Geometry: final body of the model. Coordinates: model frame, mm. Face numbers are marked on the shaded views. A direction names the side the tool comes from. Coordinates: 2 decimals unless noted, no trailing zeros. Order: outer loops, then holes, each group sorted by start corner. A loop starts at its lowest first (then second) coordinate and runs counter-clockwise, first axis right, second up. Notation, with made-up numbers: (43.25, -8.75) - (100.25, -8.75) arc R26 cw to (100.25, 13.25) - close; hole circle Ø11 at (-38.75, 81.5). An arc over 180 degrees is marked (long way). Use a Markdown table: item, result. Add a question column.
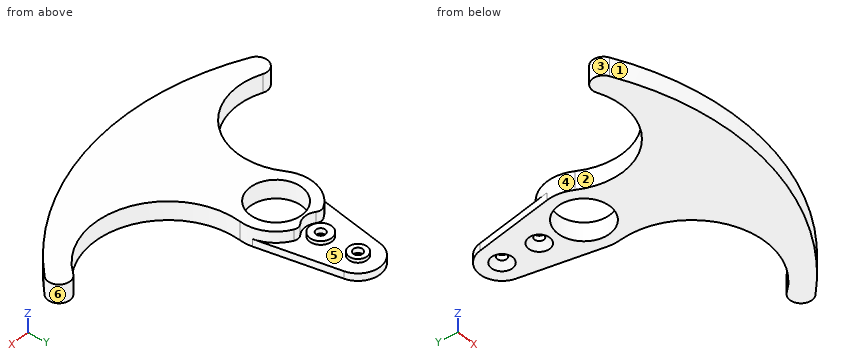
Autodesk Inventor part; units mm, degrees
ref_plane "YZ Plane" through (0, 0, 0) normal (1, 0, 0) x (0, 1, 0)
ref_plane "XZ Plane" through (0, 0, 0) normal (0, 1, 0) x (-1, 0, 0)
ref_plane "XY Plane" through (0, 0, 0) normal (0, 0, 1) x (1, 0, 0)
sketch "Sketch1" plane through (0, 0, 0) normal (0, 0, 1) x (1, 0, 0)
  line L0 (64.2929, 13) -> (99.1548, 4.0199) construction
  circle A0 centre (64.2929, 13) radius 3 construction
  circle A1 centre (64.2929, 13) radius 4.025 construction
  circle A2 centre (64.2929, 13) radius 7 construction
  arc A3 (102.6474, 8.8986) -> (63.8399, 19.9853) centre (67.7221, -39.8889) ccw construction
  circle A4 centre (99.1548, 4.0199) radius 2.5
  circle A5 centre (99.1548, 4.0199) radius 3.525
  circle A6 centre (99.1548, 4.0199) radius 6
  line L1 (64.2929, 13) -> (98.9408, 0.0186) construction
  line L2 (99.1548, 4.0199) -> (99.1548, -17.9801) construction
  line L3 (99.1548, -17.9801) -> (98.9408, 0.0186) construction
  circle A7 centre (99.1548, -17.9801) radius 10
  circle A8 centre (99.1548, -17.9801) radius 7.025
  line L4 (105.0548, 5.1108) -> (108.9881, -16.162)
  line L5 (93.2548, 5.1108) -> (89.3215, -16.162)
  line L6 (9.3628, -60) -> (214.5663, -60) construction
  arc A9 (95.4028, -0.6623) -> (65.8301, 6.1709) centre (73.5161, -27.9748) ccw construction
  line L7 (99.1548, 4.0199) -> (66.0447, -51.9827) construction
  line L8 (99.1548, 4.0199) -> (148.8226, -39.0251) construction
  circle A10 centre (67.5736, -49.3967) radius 3
  circle A11 centre (146.5507, -37.0561) radius 3
  arc A12 (68.7666, -46.6441) -> (90.4037, -22.8193) centre (75.5268, -31.046) ccw
  arc A13 (109.0459, -19.4522) -> (144.239, -35.1439) centre (128.828, -22.3964) ccw
  arc A14 (66.0447, -51.9827) -> (148.8226, -39.0251) centre (98.68, 10.4177) ccw
  circle A15 centre (99.1548, -5.9801) radius 1.25
  circle A16 centre (99.1548, -5.9801) radius 3
  circle A17 centre (99.1548, -5.9801) radius 4.25
  circle A18 centre (99.1548, 4.0199) radius 1.25
  arc A19 (103.9067, -9.1813) -> (101.7399, -9.3536) centre (102.9564, -10.9411) ccw
  arc A20 (96.5698, -9.3536) -> (94.4029, -9.1813) centre (95.3533, -10.9411) ccw
  point P0 (0, 0)
  point P1 (0, 0)
  point P2 (66.1895, -52.0583)
  point P3 (148.6808, -39.1685)
  point P4 (97.1242, -8.1885)
  point P5 (102.5276, -8.5661)
  point P6 (95.7821, -8.5661)
  dimension "d19" = 6
  dimension "d20" = 6
  dimension "d0" = 36
  dimension "d1" = 8.05
  dimension "d2" = 6
  dimension "d3" = 14
  dimension "d4" = 60
  dimension "d5" = 37
  dimension "d6" = 22
  dimension "d7" = 18
  dimension "d8" = 12
  dimension "d9" = 7.05
  dimension "d10" = 20
  dimension "d11" = 14.05
  dimension "d12" = 35
  dimension "d13" = 5
  dimension "d14" = 60
  dimension "d15" = 30.593
  dimension "d16" = 49.086
  dimension "d17" = 65.7249
  dimension "d18" = 65.0582
  dimension "d21" = 13
  dimension "d22" = 70.4193
  dimension "d23" = 17
  dimension "d24" = 20
  dimension "d29" = 2.5
  dimension "d30" = 6
  dimension "d31" = 8.5
  dimension "d32" = 2.5
  dimension "d43" = 10
  dimension "d44" = 2
  dimension "d45" = 2
extrude "Extrusion1" add sketch "Sketch1" along normal blind 5 contours A7 A20 A17 A19 | A7 A13 A11 A14 A10 A12 | A10 | A11
extrude "Extrusion3" add sketch "Sketch1" along normal blind 3 contours A4 | A16 A7 | A7 A16
extrude "Extrusion4" add sketch "Sketch1" along normal blind 2 contours A5 | A6 A17 | A6 L4 A7 A17 | A17 A7 A16 A6 | A6 A17 | A6 A17 A7 L5 | A19 A17 A7 | A17 A20 A7 | A7 A16 A17 | A7 A16 picked at (99.1548, -8.3289)
chamfer "Chamfer1" distance 1.6 angle 45 1 edges at (97.9048, -5.9801, 0)
chamfer "Chamfer2" distance 1.6 angle 45 1 edges at (97.9048, 4.0199, 0)
properties part number "ヘッケン" material "Polycarbonate, Clear"
1) Section A-A (y = -41). Return loops of the section in (x, z).
2) Section C-C (x = 138). Return loops of the section in (y, z).
3) Section B-B (y = -54). Return loops of the section in (x, z), then the cut area to 3 significant figures.
4) Draft query along Y for the marked faces 1, 2 and 3. Return one class per face: pulls with the +Y half, pulls with the -Y half, needs draft (parallel to the pull), parting line crosses it, or undercut.
5) Ray query, line 1 along X through (y, z) = (-6, 2.9); line 2 along Y through (x, z) = (90, 2.9); line 3 along Y through (x, z) = (91, 2.15). Return the intervals inside material, ascending.
6) Set-up query: the marked faces 4, 5 and 6. Return all of +Z, -Z, +X, -X, +Y, -Y with unobstructed straight access to the full face (end or side cutting, diameter ignored); none if empty.
7) Pin query (flat end, axial travel): pin 1 (2.5 mm diameter, centred on x = 98.5, y = 3, fed in from +Z); pin 2 (4 mm diameter, centred on x = 99.15, y = -5.98, fed in from -Z); pin 3 (3 mm diameter, centred on x = 84, z = 2.5, fed in from -Y). Return the tip coordinate at first contact, or that it passes through.
Values follow:
| question | item | result |
|---|---|---|
| 1 | outline | (89.31, 0) - (121.49, 0) - (121.49, 5) - (89.31, 5) - close; (136.17, 0) - (146.8, 0) - (146.8, 5) - (136.17, 5) - close |
| 2 | outline | (-48, 0) - (-40.17, 0) - (-40.17, 5) - (-48, 5) - close |
| 3 | outline | (70.23, 0) - (127.13, 0) - (127.13, 5) - (70.23, 5) - close |
| 3 | area | 284 mm² |
| 4 | face 1 | pulls with the -Y half |
| 4 | face 2 | undercut |
| 4 | face 3 | parting line crosses it |
| 5 | line 1 | x = 96.15 to 97.9, 100.4 to 102.15 |
| 5 | line 2 | y = -59.46 to -39.96, -22 to -13.96 |
| 5 | line 3 | y = -59.58 to -38.09, -24 to -12.19 |
| 6 | face 4 | +Z, -X |
| 6 | face 5 | +Z |
| 6 | face 6 | +Z, -Z |
| 7 | pin 1 | stops at z = 3 |
| 7 | pin 2 | stops at z = 0.85 |
| 7 | pin 3 | stops at y = -58.76 |
